```python
from build123d import *

# Parameters (mm, degrees)
BOSS_EXTRUDE1_DEPTH = 20
CUT_EXTRUDE1_DEPTH  = 10
SKETCH4_R           = 3
CUT_EXTRUDE2_DEPTH  = 10


with BuildPart() as part:
    # Sketch2 → Boss-Extrude1 (new body)
    with BuildSketch(Plane.XY):
        with BuildLine():
            Line((0, 2), (0, 50))
            Line((0, 50), (1, 50))
            Line((1, 50), (1, 2))
            ThreePointArc((1, 2), (1.292893219, 1.292893219), (2, 1))
            Line((2, 1), (25, 1))
            Line((25, 1), (25, 0))
            Line((25, 0), (2, 0))
            ThreePointArc((2, 0), (0.585786438, 0.585786438), (0, 2))
        make_face()
    extrude(amount=BOSS_EXTRUDE1_DEPTH)

    # Sketch3 → Cut-Extrude1 (cut)
    with BuildSketch(Plane(origin=(1, 0, 0), x_dir=(0, 0, -1), z_dir=(1, 0, 0))):
        with BuildLine():
            Line((-13, 13.5), (-13, 38.5))
            ThreePointArc((-13, 38.5), (-10, 41.5), (-7, 38.5))
            Line((-7, 38.5), (-7, 13.5))
            ThreePointArc((-7, 13.5), (-10, 10.5), (-13, 13.5))
        make_face()
    extrude(amount=-CUT_EXTRUDE1_DEPTH, mode=Mode.SUBTRACT)

    # Sketch4 → Cut-Extrude2 (cut)
    with BuildSketch(Plane(origin=(0, 1, 0), x_dir=(1, 0, 0), z_dir=(0, 1, 0))):
        with Locations((14, -10)):
            Circle(SKETCH4_R)
    extrude(amount=-CUT_EXTRUDE2_DEPTH, mode=Mode.SUBTRACT)


solid = part.part
```
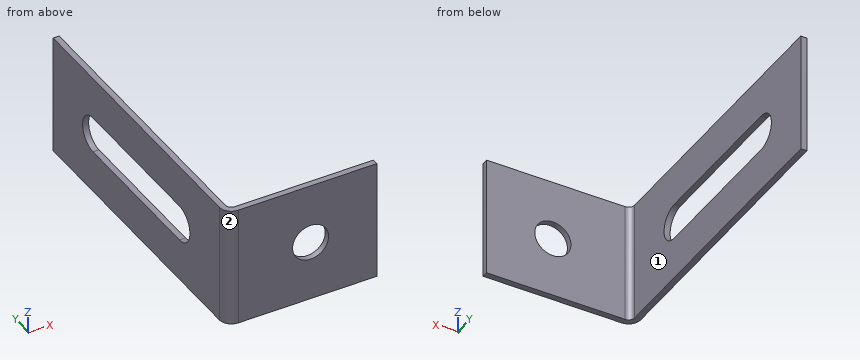
The model under review builds one solid part; all positions refer to its coordinate system, in mm. Face numbers are marked on the shaded views. A direction names the side the tool comes from. Round coordinates to 2 decimals unless told otherwise and drop trailing zeros. Write each loop counter-clockwise with the first axis right and the second up, starting at its lowest first coordinate (ties: lowest second). Pieces come first, ordered by that corner, then holes.
(1) Machinability: for the marked faces 1 and 2, which of the approach directions +Z, -Z, +X, -X, +Y, -Y give a long, thin tool a straight path to every point of the face, cutting with its end or side? Answer none if there is none.
(2) We need section B-B on y = 14. Give the boundary of the cut face in (x, z).
(3) Wall thickness on L1, parallel to Z at x = 14, y = 0.3; L2, parallel to Y at x = 6.25, z = 10.25: over which ranges is each line inside the solid? List them lowest first.
(4) We need section D-D on z = 15.25. Give the boundary of the cut face in (x, y).
(5) We need section C-C on x = 16. Give the boundary of the cut face in (y, z), and give its area (3 significant figures).
(6) Insertion check: pin 1 (5.5 mm diameter, centred on x = 14, z = 10, fed in from -Y); pin 2 (2 mm diameter, centred on x = 21.5, z = 9.5, fed in from +Y); pin 3 (10 mm diameter, centred on y = 30.5, z = 7, fed in from +X). Each pin has a flat end and moves straight along its axis. Give the tip position at first contact, or say it passes through.
(7) We need section A-A on z = 10. Give the boundary of the cut face in (x, y).
Findings below:
1. face 1: +Z, -Z, +X, +Y
1. face 2: +Z, -Z, -X, -Y
2. outline: (0, 0) - (1, 0) - (1, 7) - (0, 7) - close; (0, 13) - (1, 13) - (1, 20) - (0, 20) - close
3. L1: z = 0 to 7, 13 to 20
3. L2: y = 0 to 1
4. outline: (0, 2) arc R2 ccw to (2, 0) - (25, 0) - (25, 1) - (2, 1) arc R1 cw to (1, 2) - (1, 50) - (0, 50) - close
5. outline: (0, 0) - (1, 0) - (1, 7.76) - (0, 7.76) - close; (0, 12.24) - (1, 12.24) - (1, 20) - (0, 20) - close
5. area: 15.5 mm2
6. pin 1: passes through
6. pin 2: stops at y = 1
6. pin 3: stops at x = 1
7. outline: (0, 2) arc R2 ccw to (2, 0) - (11, 0) - (11, 1) - (2, 1) arc R1 cw to (1, 2) - (1, 10.5) - (0, 10.5) - close; (0, 41.5) - (1, 41.5) - (1, 50) - (0, 50) - close; (17, 0) - (25, 0) - (25, 1) - (17, 1) - close
